For this review, take the finished solid that the model builds, in its own axes (mm). Coordinates: 2 decimals unless noted, no trailing zeros. Write each loop counter-clockwise with the first axis right and the second up, starting at its lowest first coordinate (ties: lowest second). Pieces come first, ordered by that corner, then holes. Notation, with made-up numbers: (-13.75, -21) -> (45.25, -21) arc R21 ccw to (45.25, -10) -> close; hole circle Ø8 at (83.5, -1.5). An arc over 180 degrees is marked (long way). Put each result on its own line as item: value. Start each with the question number.
Item 1: Consider section B-B on x = 0.5. Give the boundary of the cut face in (y, z), and give its area (3 significant figures).
Item 2: The part is to be moulded in two halves that separate along Y. For faces 1 (the flat face through (0, 0, 4.4)), 2 (the flat face through (0, 3.65, 2)), 3 (the flat face through (-3.65, 0, 2)), say which applies: +Y half, -Y half, draft (parallel to the pull), parting line (faces both ways), or undercut.
Item 3: To check wall thickness, follow L1, parallel to Z at x = -2.5, y = 2. State the ranges of the line that lie inside material, in increasing order.
Item 4: Consider section A-A on y = 0. Give the boundary of the cut face in (x, z).
```python
from build123d import *

# Parameters (mm, degrees)
SKETCH_1_W               = 7.3
SKETCH_1_H               = 7.3
EXTRUDE_1_DEPTH          = 4.5
FILLET_1_R               = 0.5
SKETCH_2_R               = 2.7
CUT_EXTRUDE_1_DEPTH      = 0.1
CUT_EXTRUDE_2_DEPTH      = 0.1
PATTERN_CIRCULAR_1_COUNT = 4


with BuildPart() as part:
    # Эскиз1 → Бобышка-Вытянуть1 (new body)
    with BuildSketch(Plane.XY):
        Rectangle(SKETCH_1_W, SKETCH_1_H)
    extrude(amount=EXTRUDE_1_DEPTH)

    # Скругление1
    fillet_1_edges = [part.edges().sort_by_distance(p)[0] for p in [
        (3.65, -3.65, 2.25),
        (-3.65, -3.65, 2.25),
        (-3.65, 3.65, 2.25),
        (3.65, 3.65, 2.25),
    ]]
    fillet(fillet_1_edges, radius=FILLET_1_R)

    # Эскиз2 → Вырез-Вытянуть1 (cut)
    with BuildSketch(Plane.XY.offset(4.5)):
        Circle(SKETCH_2_R)
    extrude(amount=-CUT_EXTRUDE_1_DEPTH, mode=Mode.SUBTRACT)

    # Эскиз3 → Вырез-Вытянуть2 (cut)
    with BuildSketch(Plane.XY.offset(4.5)):
        Polygon((-2.799540108, 1.993438378), (-2.269210022, 1.463108292), (-1.463108292, 2.269210022), (-1.993438378, 2.799540108), align=None)
    cut_extrude_2 = extrude(amount=-CUT_EXTRUDE_2_DEPTH, mode=Mode.SUBTRACT)

    # Круговой массив1: Вырез-Вытянуть2 ×4 about axis
    pattern_circular_1_axis = Axis((0, 0, 0), (0, 0, 1))
    for i in range(1, PATTERN_CIRCULAR_1_COUNT):
        add(cut_extrude_2.rotate(pattern_circular_1_axis, i * 360 / PATTERN_CIRCULAR_1_COUNT), mode=Mode.SUBTRACT)


solid = part.part
```
Return value:
1. outline: (-3.65, 0) -> (3.65, 0) -> (3.65, 4.5) -> (2.65, 4.5) -> (2.65, 4.4) -> (-2.65, 4.4) -> (-2.65, 4.5) -> (-3.65, 4.5) -> close
1. area: 32.3 mm^2
2. face 1: undercut
2. face 2: +Y half
2. face 3: draft
3. L1: 0 to 4.4
4. outline: (-3.65, 0) -> (3.65, 0) -> (3.65, 4.5) -> (2.7, 4.5) -> (2.7, 4.4) -> (-2.7, 4.4) -> (-2.7, 4.5) -> (-3.65, 4.5) -> close
